Solid Edge part; units mm, degrees
sketch "Sketch1" plane through (0, 0, 0) normal (0, 0, 1) x (1, 0, 0)
  line L0 (12.7, -12.7) -> (8.0776, 0)
  line L1 (8.0776, 0) -> (8.0776, 25.4)
  line L2 (8.0776, 25.4) -> (-8.0776, 25.4)
  line L3 (-8.0776, 25.4) -> (-8.0776, 0)
  line L4 (-12.7, -12.7) -> (-8.0776, 0)
  line L5 (-12.7, -12.7) -> (12.7, -12.7)
extrude "Protrusion1" add sketch "Sketch1" against normal blind 50.8
sketch "Sketch2" plane through (0, 25.4, -25.4) normal (0, 1, 0) x (0, 0, -1)
  circle A0 centre (25.4, 0) radius 12.7
extrude "ExtrudedCutout_1" cut sketch "Sketch2" against normal blind 20.32
sketch "Sketch3" plane through (0, 25.4, -25.4) normal (0, 1, 0) x (0, 0, -1)
  circle A0 centre (25.4, 0) radius 25.4
extrude "ExtrudedCutout_2" cut sketch "Sketch3" against normal blind 15.24
sketch "Sketch4" plane through (0, 25.4, -25.4) normal (0, 1, 0) x (0, 0, -1)
  circle A0 centre (25.4, 0) radius 41.275
extrude "ExtrudedCutout_3" cut sketch "Sketch4" against normal blind 10.16
fillet "Round_1" radius 1.27 6 edges at (8.0776, 20.32, -10.3231) (-8.0776, 20.32, -10.3231) (8.0776, 12.7, -26.7186) (-8.0776, 12.7, -26.7186) (8.0776, 7.62, -40.9999) (-8.0776, 7.62, -40.9999)
hole "Hole_1" at (-0.0844, 15.24, -17.1073) direction (0, -1, 0) diameter 6.2484 end up to next counterbore diameter 9.9212 counterbore depth 5.08
hole "Hole_2" at (-0.011, 10.16, -31.6589) direction (0, -1, 0) diameter 6.2484 end up to next counterbore diameter 9.9212 counterbore depth 5.08
hole "Hole1" at (0, 10.16, -45.064) direction (0, -1, 0) diameter 6.2484 end up to next counterbore diameter 9.9212 counterbore depth 5.08
Verification items for the finished model (mm, model axes). A direction names the side the tool comes from. Give positions to 0.01 mm unless a question says otherwise; leave off trailing zeros. Write each loop counter-clockwise with the first axis right and the second up, starting at its lowest first coordinate (ties: lowest second). Pieces come first, ordered by that corner, then holes.
(1) Cross-section at A-A (y = -1). Enter the section's corners in (x, z), plus the area to 3 significant figures.
(2) Material ranges on line 1 (Y direction, x = -5, z = -31.5); line 2 (Y direction, x = 3.75, z = -33); line 3 (Z direction, x = -0.5, y = 4), recorded low to high.
(3) Access from +Z, -Z, +X, -X, +Y, -Y to the whole of each face (thin tool, end or side, straight path). Record for faces 1 (the face through (0, -12.7, -25)), 2 (the face through (1.816, 12.664, -12.525)), 3 (the face through (-7.43, 7.66, -39.71)).
(4) Mould release check, pull along X, two halves, no side actions. Record for faces 4 (the face through (-8.078, 10, -19)), 5 (the face through (3.2, 10.16, -17.2)), 6 (the face through (0, 7, 0)), 7 (the face through (-0.1, 7.7, -38.1)): +X half, -X half, draft (parallel to the pull), parting line (faces both ways), or undercut.
(5) Cross-section at B-B (z = -4.5). Enter the section's corners in (x, y), plus the area to 3 significant figures.
(6) Gauge pin test, flat ends, axial feed: pin 1 (3.5 mm diameter, centred on x = -0.08, z = -17.11, fed in from -Y); pin 2 (10 mm diameter, centred on x = -8.5, z = -27, fed in from +Y); pin 3 (6.5 mm diameter, centred on x = -3.5, z = -45, fed in from +Y); pin 4 (10 mm diameter, centred on y = -2.5, z = -31.5, fed in from -X). Record the tip position at first contact, or that the pin passes through.
(7) Cross-section at C-C (x = -2.25). State how many separate pieces and enclosed holes the cut face has, plus the area to 3 significant figures.
(8) Cross-section at D-D (y = 20). Enter the section's corners in (x, z) (3 decimals).
Worked out:
1. outline: (-8.44, -50.8) - (8.44, -50.8) - (8.44, 0) - (-8.44, 0) - close; hole circle Ø6.25 at (-0.08, -17.11); hole circle Ø6.25 at (-0.01, -31.66); hole circle Ø6.25 at (0, -45.06)
1. area: 766 mm2
2. line 1: y = -12.7 to 10.16
2. line 2: y = -12.7 to 5.08
2. line 3: z = -50.8 to -48.15, -41.98 to -34.74, -28.57 to -20.2, -14.01 to 0
3. face 1: +Z, -Z, +X, -X, -Y
3. face 2: +Y
3. face 3: -Z, +Y
4. face 4: -X half
4. face 5: undercut
4. face 6: draft
4. face 7: undercut
5. outline: (-12.7, -12.7) - (12.7, -12.7) - (8.08, 0) - (8.08, 25.4) - (-8.08, 25.4) - (-8.08, 0) - close
5. area: 674 mm2
6. pin 1: passes through
6. pin 2: stops at y = 15.24
6. pin 3: stops at y = 5.08
6. pin 4: stops at x = -10.81
7. separate pieces: 4
7. enclosed holes: 0
7. area: 977 mm2
8. outline: (-8.078, -8.803) arc R1.27 ccw to (-6.604, -10.057) arc R41.275 cw to (6.604, -10.057) arc R1.27 ccw to (8.078, -8.803) - (8.078, 0) - (-8.078, 0) - close
